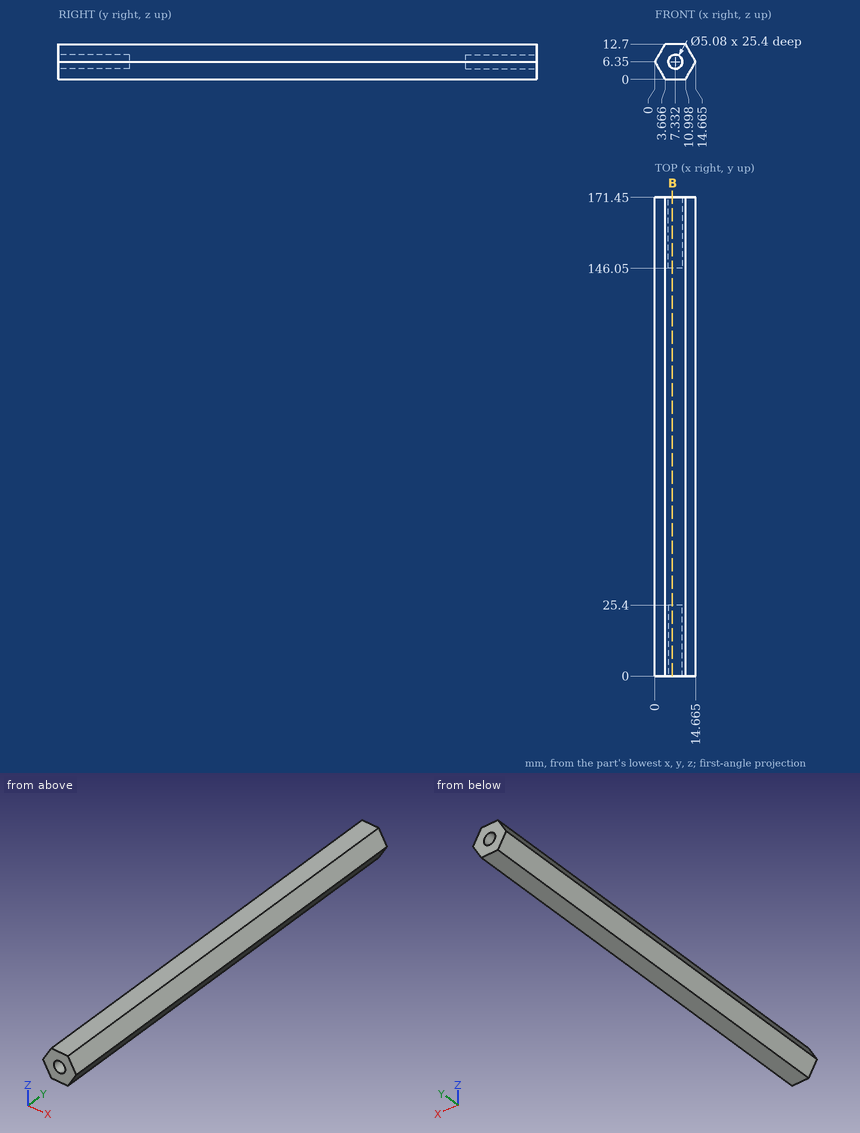
Design review of the part shown in the three views and the two pictorial views. Dimensions are in mm from the part's minimum x, y and z. Coordinates: 2 decimals unless noted, no trailing zeros. Write each loop counter-clockwise with the first axis right and the second up, starting at its lowest first coordinate (ties: lowest second). Pieces come first, ordered by that corner, then holes.
1) To check wall thickness, follow probe 1 along Y at (x, z) = (9.75, 7); probe 2 along Z at (x, y) = (13.75, 58) (1 decimal); probe 3 along Z at (x, y) = (13.5, 105) (1 decimal). State the ranges of each line that lie inside material, in increasing order.
2) We need section B-B on x = 6.25. State the section outline as (y, z) points, then the cut area to 3 significant figures.
3) Clearance check with flat-ended pins moving along their axes: pin 1 Ø4.5 at (x, z) = (7.33, 6.35) entering from +Y; pin 2 Ø1 at (y, z) = (67, 9) entering from -X; pin 3 Ø1 at (y, z) = (67.5, 7) entering from -X. State where each tip first meets the part, or that it passes through.
Answer list:
1. probe 1: y = 25.4 to 146.05
1. probe 2: z = 4.8 to 7.9
1. probe 3: z = 4.3 to 8.4
2. outline: (0, 0) - (171.45, 0) - (171.45, 4.05) - (146.05, 4.05) - (146.05, 8.65) - (171.45, 8.65) - (171.45, 12.7) - (0, 12.7) - (0, 8.65) - (25.4, 8.65) - (25.4, 4.05) - (0, 4.05) - close
2. area: 1,940 mm2
3. pin 1: stops at y = 146.05
3. pin 2: stops at x = 1.24
3. pin 3: stops at x = 0.09
